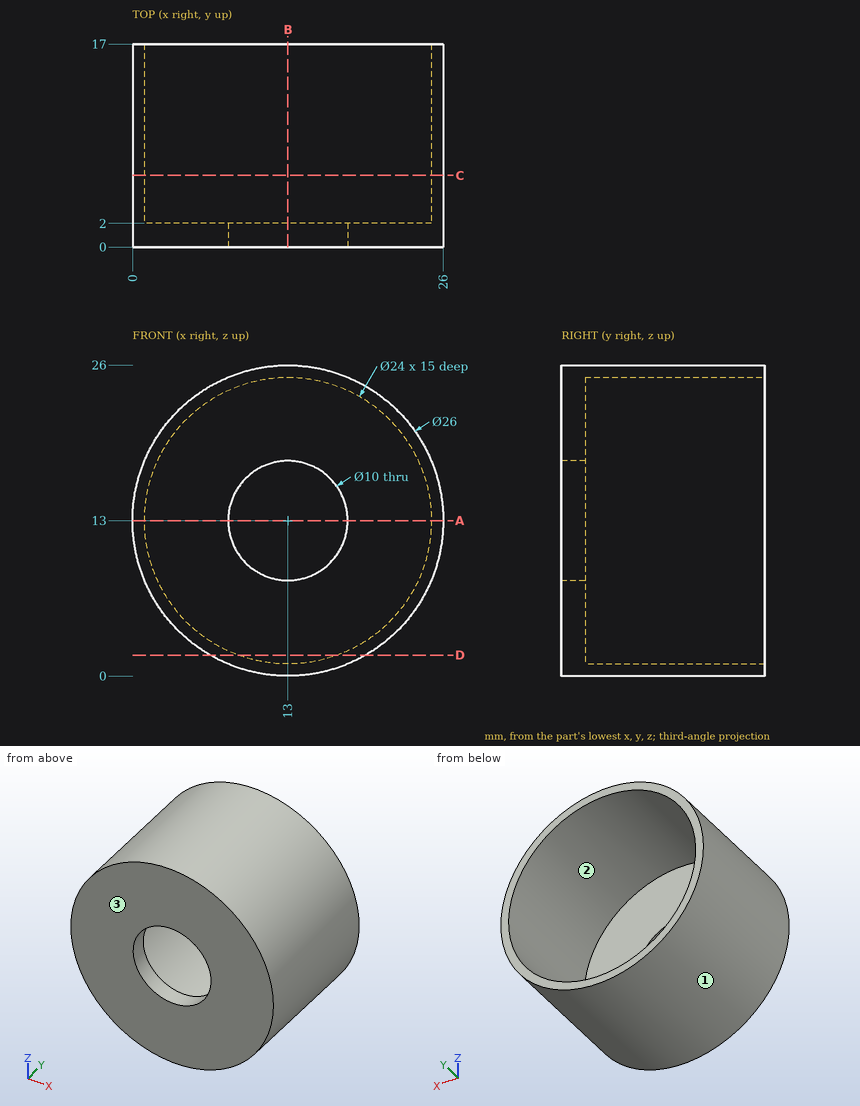
For this review, use the dimensioned drawing (mm, ordinates from the lowest corner) and the shaded views. Round coordinates to 2 decimals unless told otherwise and drop trailing zeros. Write each loop counter-clockwise with the first axis right and the second up, starting at its lowest first coordinate (ties: lowest second). Pieces come first, ordered by that corner, then holes. Notation, with made-up numbers: (19.5, 66.5) -> (35.5, 66.5) arc R26 cw to (35.5, 85.5) -> close; hole circle Ø1 at (73.25, -40). An arc over 180 degrees is marked (long way). Use one line per item in the form item = value.
Q1. The part is to be moulded in two halves that separate along Z. For the marked faces 1, 2 and 3, say which applies: released by +Z, released by -Z, zero draft, split by the parting line, or undercut.
Resolved:
face_1 = split by the parting line
face_2 = undercut
face_3 = zero draft
Q2. Consider section D-D (z = 1.75). State the section outline as (x, y) points.
Resolved:
outline = (6.49, 0) -> (19.51, 0) -> (19.51, 17) -> (17.18, 17) -> (17.18, 2) -> (8.82, 2) -> (8.82, 17) -> (6.49, 17) -> close
Q3. To check wall thickness, follow probe 1 along X at (y, z) = (0.85, 13); probe 2 along X at (y, z) = (13, 9); probe 3 along Y at (x, z) = (2.75, 16.5). State the ranges of each line that lie inside material, in increasing order. Write a range as from..to.
Resolved:
probe_1 = 0..8, 18..26
probe_2 = 0.63..1.69, 24.31..25.37
probe_3 = 0..2
Q4. Consider section A-A (z = 13). State the section outline as (x, y) points.
Resolved:
outline = (0, 0) -> (8, 0) -> (8, 2) -> (1, 2) -> (1, 17) -> (0, 17) -> close; (18, 0) -> (26, 0) -> (26, 17) -> (25, 17) -> (25, 2) -> (18, 2) -> close
Q5. Consider section C-C (y = 6). State the section outline as (x, z) points.
Resolved:
outline = circle Ø26 at (13, 13); hole circle Ø24 at (13, 13)
Q6. Clearance check with flat-ended pins moving along their axes: pin 1 Ø4 at (y, z) = (5, 10.5) entering from +X; pin 2 Ø1 at (x, y) = (12, 3.5) entering from +Z; pin 3 Ø12 at (x, z) = (17, 15) entering from +Y. State where each tip first meets the part, or that it passes through.
Resolved:
pin_1 = 25.99
pin_2 = 25.99
pin_3 = 2
Q7. Consider section B-B (x = 13). State the section outline as (y, z) points, then the cut area to 3 significant figures.
Resolved:
outline = (0, 0) -> (17, 0) -> (17, 1) -> (2, 1) -> (2, 8) -> (0, 8) -> close; (0, 18) -> (2, 18) -> (2, 25) -> (17, 25) -> (17, 26) -> (0, 26) -> close
area = 62.0 mm²
